```python
from build123d import *

# Parameters (mm, degrees)
SALIENTE_EXTRUIR1_DEPTH = 10
CROQUIS6_R              = 17.5
CORTAR_EXTRUIR5_DEPTH   = 203.484567313
CROQUIS7_R              = 2.5
CORTAR_EXTRUIR6_DEPTH   = 10
SKETCH1_W               = 10
SKETCH1_H               = 60
BOSS_EXTRUDE1_DEPTH     = 50
SKETCH2_R               = 2.5
CUT_EXTRUDE1_DEPTH      = 10
SKETCH5_R               = 2.5
CUT_EXTRUDE2_DEPTH      = 252.992063367
SKETCH6_R               = 17.5
SKETCH6_R_2             = 6.5
BOSS_EXTRUDE2_DEPTH     = 10
SKETCH7_R               = 3.25
CUT_EXTRUDE3_DEPTH      = 10
CIRPATTERN1_COUNT       = 6


with BuildPart() as part:
    # Croquis1 → Saliente-Extruir1 (new body)
    with BuildSketch(Plane.XY):
        with BuildLine():
            Line((200, 30), (200, -30))
            Line((200, -30), (0, -30))
            ThreePointArc((0, -30), (-30, 0), (0, 30))
            Line((0, 30), (200, 30))
        make_face()
    extrude(amount=SALIENTE_EXTRUIR1_DEPTH)

    # Croquis6 → Cortar-Extruir5 (cut, through all)
    with BuildSketch(Plane.XY.offset(10)):
        Circle(CROQUIS6_R)
    extrude(amount=-CORTAR_EXTRUIR5_DEPTH, mode=Mode.SUBTRACT)

    # Croquis7 → Cortar-Extruir6 (cut)
    with BuildSketch(Plane.XY.offset(10)):
        with Locations((195, 22.5)):
            Circle(CROQUIS7_R)
        with Locations((195, -22.5)):
            Circle(CROQUIS7_R)
    extrude(amount=-CORTAR_EXTRUIR6_DEPTH, mode=Mode.SUBTRACT)

    # Sketch1 → Boss-Extrude1 (add)
    with BuildSketch(Plane(origin=(200, 0, 0), x_dir=(0, 0, -1), z_dir=(1, 0, 0))):
        with Locations((-5, 0)):
            Rectangle(SKETCH1_W, SKETCH1_H)
    extrude(amount=BOSS_EXTRUDE1_DEPTH)

    # Sketch2 → Cut-Extrude1 (cut)
    with BuildSketch(Plane(origin=(250, 0, 0), x_dir=(0, 0, -1), z_dir=(1, 0, 0))):
        with Locations((-5, 0)):
            Circle(SKETCH2_R)
        with Locations((-5, 20)):
            Circle(SKETCH2_R)
        with Locations((-5, -20)):
            Circle(SKETCH2_R)
    extrude(amount=-CUT_EXTRUDE1_DEPTH, mode=Mode.SUBTRACT)

    # Sketch5 → Cut-Extrude2 (cut, through all)
    with BuildSketch(Plane.XY.offset(10)):
        with Locations((230, -22.5)):
            Circle(SKETCH5_R)
    extrude(amount=-CUT_EXTRUDE2_DEPTH, mode=Mode.SUBTRACT)

    # Sketch6 → Boss-Extrude2 (add)
    with BuildSketch(Plane.XY.offset(10)):
        Circle(SKETCH6_R)
        Circle(SKETCH6_R_2, mode=Mode.SUBTRACT)
    extrude(amount=-BOSS_EXTRUDE2_DEPTH)

    # Sketch7 → Cut-Extrude3 (cut)
    with BuildSketch(Plane.XY.offset(10)):
        with Locations((0, 20)):
            Circle(SKETCH7_R)
    cut_extrude3 = extrude(amount=-CUT_EXTRUDE3_DEPTH, mode=Mode.SUBTRACT)

    # CirPattern1: Cut-Extrude3 ×6 about axis
    cirpattern1_axis = Axis((0, 0, 0), (0, 0, 1))
    for i in range(1, CIRPATTERN1_COUNT):
        add(cut_extrude3.rotate(cirpattern1_axis, i * 360 / CIRPATTERN1_COUNT), mode=Mode.SUBTRACT)


solid = part.part
```
Here's how the part is built. I have some questions about the finished solid (model axes, mm). A direction names the side the tool comes from. Give positions to 0.01 mm unless a question says otherwise; leave off trailing zeros. Loops run counter-clockwise (first coordinate to the right, second up) from the corner with the lowest first, then second, coordinate; pieces in that order, holes last. Notation, with made-up numbers: M 76,60.25 L 107,60.25 A14 cw 107,84.25 Z; hole C 9,21 d11. An arc over 180 degrees is marked long. Use one line per item in the form item = value. Start each with the question number.
Q1. If we section it at B-B (z = 6): State how many separate pieces and enclosed holes the cut face has, then the cut area to 3 significant figures.
Q2. Thinking about a two-plate mould opening in X: for faces 1 (the cylindrical face through (245.07, 22.11, 3.66)), 2 (the cylindrical face through (19.716, 7.803, 5.07)), 3 (the cylindrical face through (-19.716, -7.803, 5.07)), 4 (the flat face through (240, -20, 5)), which applies, +X half, -X half, draft (parallel to the pull), parting line (faces both ways), or undercut?
Q3. I need wall thicknesses on line 1 along Y through (x, z) = (0, 4); line 2 along Y through (x, z) = (245.5, 5); line 3 along X through (y, z) = (-11.5, 1.25). Which ranges of each line are inside material? Lowest first, please.
Q4. Will these pins go through, and if not, where does the flat tip stop? pin 1 Ø2 at (x, y) = (64.5, 21) entering from -Z; pin 2 Ø6 at (x, y) = (0, -20) entering from -Z; pin 3 Ø3 at (y, z) = (-20, 5) entering from +X.
Q5. If we section it at A-A (y = 0): Write out the boundary of the cut face in (x, z).
Q6. Which directions (+Z, -Z, +X, -X, +Y, -Y) give clear straight access to the entire face, cutting with the end or side of a thin tool? Please do faces 5 (the cylindrical face through (245.07, 0.751, 2.615)), 6 (the flat face through (250, 0, 8)).
Taken from the geometry:
q1.separate_pieces = 1
q1.enclosed_holes = 10
q1.area = 15,900 mm^2
q2.face_1 = draft
q2.face_2 = undercut
q2.face_3 = undercut
q2.face_4 = +X half
q3.line_1 = -30 to -23.25, -16.75 to -6.5, 6.5 to 16.75, 23.25 to 30
q3.line_2 = -30 to -22.5, -17.5 to -2.5, 2.5 to 17.5, 22.5 to 30
q3.line_3 = -27.71 to -20.2, -14.44 to 14.44, 20.2 to 250
q4.pin_1 = 0
q4.pin_2 = through
q4.pin_3 = 240
q5.outline = M -30,0 L -6.5,0 L -6.5,10 L -30,10 Z; M 6.5,0 L 250,0 L 250,2.5 L 240,2.5 L 240,7.5 L 250,7.5 L 250,10 L 6.5,10 Z
q6.face_5 = +X
q6.face_6 = +Z, -Z, +X, +Y, -Y
